Here's how the part is built. I have some questions about the finished solid (model axes, mm). Coordinates: 2 decimals unless noted, no trailing zeros. Order: outer loops, then holes, each group sorted by start corner. A loop starts at its lowest first (then second) coordinate and runs counter-clockwise, first axis right, second up. Notation, with made-up numbers: (5, 44) - (61, 44) arc R30 ccw to (61, 70) - close; hole circle Ø10 at (-17.75, 32). An arc over 180 degrees is marked (long way). Answer as CSV lines item,"result". Start each with the question number.
Q1. I need wall thicknesses on line 1 (Y direction, x = 0, z = -15); line 2 (X direction, y = -12, z = -12); line 3 (X direction, y = -13, z = 11.5). Which ranges of each line are inside material? Lowest first, please.
Q2. For pin 1 Ø10 at (x, y) = (-11.5, 1) entering from +Z; pin 2 Ø8 at (y, z) = (-23.5, 0) entering from -X; pin 3 Ø9.5 at (y, z) = (-20, -6) entering from -X; pin 4 Ø3 at (y, z) = (10, -9) entering from -X, each with a flat end and sliding along its axis, tell me the tip position at first contact or that it passes through.
Q3. Suppose I cut it at A-A (z = 0). Please give me the cut outline in (x, y), then the cut area to 3 significant figures.
Autodesk Inventor part; units mm, degrees
ref_plane "YZ Plane" through (0, 0, 0) normal (1, 0, 0) x (0, 1, 0)
ref_plane "XZ Plane" through (0, 0, 0) normal (0, 1, 0) x (-1, 0, 0)
ref_plane "XY Plane" through (0, 0, 0) normal (0, 0, 1) x (1, 0, 0)
sketch "Sketch1" plane through (0, 0, 0) normal (0, 0, 1) x (1, 0, 0)
  circle A0 centre (0, 0) radius 20
  circle A1 centre (0, 0) radius 23.5
  line L0 (23.5, 0) -> (23, 0)
  line L1 (23, 0) -> (23, -36.2)
  line L2 (23, -36.2) -> (23.5, -36.2)
  line L3 (23.5, -36.2) -> (23.5, 0)
  circle A2 centre (0, 0) radius 23
  circle A3 centre (0, 0) radius 22.5
  circle A4 centre (0, 0) radius 22
  circle A5 centre (0, 0) radius 21.5
  circle A6 centre (0, 0) radius 21
  circle A7 centre (0, 0) radius 20.5
  point P0 (23, -4.8218)
  point P1 (0, -23.5)
  dimension "d0" = 40
  dimension "d1" = 47
  dimension "d2" = 0.5
  dimension "d3" = 0.5
  dimension "d4" = 0.5
  dimension "d5" = 0.5
  dimension "d6" = 0.5
  dimension "d7" = 0.5
  dimension "d58" = 12.7
extrude "Extrusion1" add sketch "Sketch1" along normal mid plane 31.75 contours A7
chamfer "Chamfer3" distance 0.1 angle 45 4 edges at (-20.5, 0, 15.875) (-20, 0, 15.875) (-20.5, 0, -15.875) (-20, 0, -15.875)
extrude "Extrusion2" add sketch "Sketch1" along normal mid plane 31.75 contours A6
chamfer "Chamfer4" distance 0.1 angle 45 4 edges at (-21, 0, 15.875) (-21, 0, -15.875) (-20.5, 0, 15.875) (-20.5, 0, -15.775)
extrude "Extrusion3" add sketch "Sketch1" along normal mid plane 31.75 contours A5
chamfer "Chamfer5" distance 0.1 angle 45 4 edges at (-21.5, 0, 15.875) (-21, 0, 15.875) (-21.5, 0, -15.875) (-21, 0, -15.875)
extrude "Extrusion4" add sketch "Sketch1" along normal mid plane 31.75 contours A4
chamfer "Chamfer6" distance 0.1 angle 45 4 edges at (-22, 0, 15.875) (-21.5, 0, 15.875) (-22, 0, -15.875) (-21.5, 0, -15.875)
extrude "Extrusion5" add sketch "Sketch1" along normal mid plane 31.75 contours A3
chamfer "Chamfer7" distance 0.1 angle 45 4 edges at (-22.5, 0, 15.875) (-22, 0, 15.875) (-22.5, 0, -15.875) (-22, 0, -15.875)
extrude "Extrusion6" add sketch "Sketch1" along normal mid plane 31.75 contours A2
chamfer "Chamfer8" distance 0.1 angle 45 4 edges at (-23, 0, 15.875) (-22.5, 0, 15.875) (-23, 0, -15.875) (-22.5, 0, -15.875)
extrude "Extrusion7" add sketch "Sketch1" along normal mid plane 31.75 contours L0 L1 A1 | L3 L2 L1 A1 | A1 L1 L0
fillet "Fillet1" radius 12.7 2 edges at (23.25, -36.2, 15.875) (23.25, -36.2, -15.875)
chamfer "Chamfer9" distance 0.1 angle 45 9 edges at (23.5, -11.75, 15.875) (-23.3747, 2.4238, 15.875) (23.5, -32.4803, 12.1553) (23.5, -11.75, -15.875) (-23.3747, 2.4238, -15.875) (-23, 0, 15.875) (23, -14.1609, 15.875) (23, -32.4803, 12.1553) (23, -14.1609, -15.875)
sketch "Sketch2" plane through (23.5, -23.5, 15.775) normal (1, 0, 0) x (0, 0, -1)
  line L0 (0, 0) -> (0, 23.5)
  arc A0 (0, 0) -> (12.6, -12.6) centre (12.6, 0) ccw
  line L1 (18.95, -12.6) -> (12.6, -12.6)
  arc A1 (18.95, -12.6) -> (31.55, 0) centre (18.95, 0) ccw
  line L2 (31.55, 23.5) -> (31.55, 0)
  line L3 (31.55, 23.5) -> (0, 23.5)
  line L4 (12.6, 0) -> (18.95, 0)
  point P0 (15.775, 23.5)
  point P1 (15.775, 0)
hole "Hole1" at (23.5, -23.5, 0) direction (-1, 0, 0) diameter 4.9784 depth 0.5
equation "\"d3\" = d2"
equation "\"d13\" = Thickness"
equation "\"d18\" = Thickness"
equation "\"d20\" = Thickness"
equation "\"d22\" = Thickness"
equation "\"d24\" = Thickness"
equation "\"d26\" = Thickness"
properties part number "TTB Elevator Constant Force Spring" material "Steel"
Here are the results:
1,line 1,"y = -23.5 to -20, 20 to 23.5"
1,line 2,"x = -20.21 to -16, 16 to 20.21, 23 to 23.5"
1,line 3,"x = -19.58 to -15.2, 15.2 to 19.58, 23 to 23.5"
2,pin 1,"passes through"
2,pin 2,"stops at x = -13.11"
2,pin 3,"stops at x = -17.88"
2,pin 4,"stops at x = -21.91"
3,outline,"(23, -36.1) - (23.1, -36.2) - (23.4, -36.2) - (23.5, -36.1) - (23.5, -25.99) - (23, -25.99) - close; (23, -21.01) - (23.5, -21.01) - (23.5, 0) arc R23.5 ccw (long way) to (23, -4.82) - close; hole circle Ø40 at (0, 0)"
3,area,"492 mm²"
